from build123d import *

# Parameters (mm, degrees)
SKETCH_1_W      = 450
SKETCH_1_H      = 400
EXTRUDE_1_DEPTH = 50
SKETCH_2_W      = 450
SKETCH_2_H      = 30
EXTRUDE_2_DEPTH = 400
SKETCH_3_W      = 40
SKETCH_3_H      = 40
EXTRUDE_3_DEPTH = 450
SKETCH_4_W      = 40
SKETCH_4_H      = 40
EXTRUDE_4_DEPTH = 450
SKETCH_5_W      = 40
SKETCH_5_H      = 40
EXTRUDE_5_DEPTH = 450
SKETCH_6_W      = 40
SKETCH_6_H      = 40
EXTRUDE_6_DEPTH = 450


with BuildPart() as part:
    # Sketch 1 → Extrude 1 (new body)
    with BuildSketch(Plane.XY):
        Rectangle(SKETCH_1_W, SKETCH_1_H)
    extrude(amount=EXTRUDE_1_DEPTH)

    # Sketch 2 → Extrude 2 (add)
    with BuildSketch(Plane(origin=(0, 0, 0), x_dir=(-1, 0, 0), z_dir=(0, 0, -1))):
        Rectangle(SKETCH_2_W, SKETCH_2_H)
    extrude(amount=EXTRUDE_2_DEPTH)

    # Sketch 4 → Extrude 4 (add)
    with BuildSketch(Plane.XY):
        with Locations((-180, 150)):
            Rectangle(SKETCH_4_W, SKETCH_4_H)
    extrude(amount=EXTRUDE_4_DEPTH)



with BuildPart() as body_2:
    # Sketch 3 → Extrude 3 (new body)
    with BuildSketch(Plane.XZ.offset(15)):
        with Locations((180, 150)):
            Rectangle(SKETCH_3_W, SKETCH_3_H)
    extrude(amount=EXTRUDE_3_DEPTH)


with BuildPart() as part_1:
    add(part.part)

    add(body_2.part)  # Extrude 5 merges body 2
    # Sketch 5 → Extrude 5 (add)
    with BuildSketch(Plane.XY):
        with Locations((180, -150)):
            Rectangle(SKETCH_5_W, SKETCH_5_H)
    extrude(amount=EXTRUDE_5_DEPTH)

    # Sketch 6 → Extrude 6 (add)
    with BuildSketch(Plane.XY):
        with Locations((-180, -150)):
            Rectangle(SKETCH_6_W, SKETCH_6_H)
    extrude(amount=EXTRUDE_6_DEPTH)


solid = part_1.part
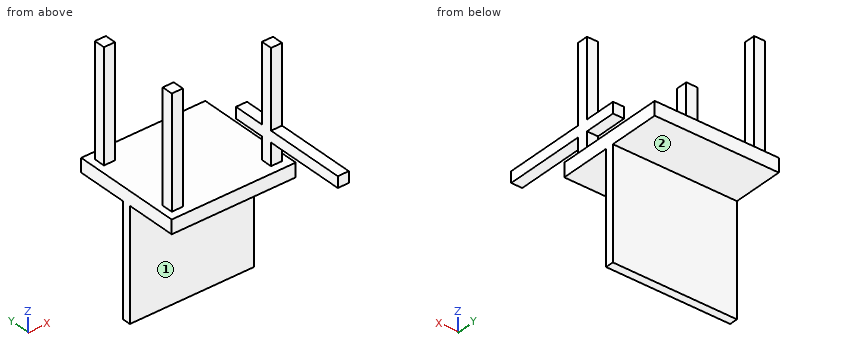
Can you work these out from the model? Positions are in its coordinate system, mm. Face numbers are marked on the shaded views. A direction names the side the tool comes from. Coordinates: 2 decimals unless noted, no trailing zeros. Order: outer loops, then holes, each group sorted by start corner. A loop starts at its lowest first (then second) coordinate and runs counter-clockwise, first axis right, second up. Notation, with made-up numbers: M -22.5,82 L 22.5,82 A15 cw 22.5,89 Z; hole C -35.75,89 d6. An arc over 180 degrees is marked long. Write item = value, one per line.
(1) Suppose I cut it at B-B on z = 252. Please give me the cut outline in (x, y).
Results are:
outline = M -200,-170 L -160,-170 L -160,-130 L -200,-130 Z; M -200,130 L -160,130 L -160,170 L -200,170 Z; M 160,-170 L 200,-170 L 200,-130 L 160,-130 Z
(2) Suppose I cut it at D-D on y = -147.5. Please give me the cut outline in (x, z), plus the area to 3 significant figures.
Results are:
outline = M -225,0 L 225,0 L 225,50 L 200,50 L 200,450 L 160,450 L 160,50 L -160,50 L -160,450 L -200,450 L -200,50 L -225,50 Z
area = 54,500 mm2
(3) I need wall thicknesses on line 1 along X through (y, z) = (-154, 200.5); line 2 along Z through (x, y) = (-7.5, -143.5); line 3 along Z through (x, y) = (105, 3). Which ranges of each line are inside material? Lowest first, please. Write a range as [from, to].
Results are:
line_1 = [-200, -160], [160, 200]
line_2 = [0, 50]
line_3 = [-400, 50]
(4) For pin 1 Ø12 at (x, z) = (176, 304) entering from -Y; pin 2 Ø1 at (x, z) = (-114.5, -145.5) entering from -Y; pin 3 Ø20 at (x, z) = (-184.5, 294.5) entering from +Y, each with a flat end and sliding along its axis, tell me the tip position at first contact or that it passes through.
Results are:
pin_1 = -170
pin_2 = -15
pin_3 = 170
(5) Suppose I cut it at C-C on x = 35. Please give me the cut outline in (y, z), plus the area to 3 significant figures.
Results are:
outline = M -200,0 L -15,0 L -15,-400 L 15,-400 L 15,0 L 200,0 L 200,50 L -200,50 Z
area = 32,000 mm2
(6) Suppose I cut it at A-A on y = -66. Please give me the cut outline in (x, z).
Results are:
outline = M -225,0 L 225,0 L 225,50 L -225,50 Z; M 160,130 L 200,130 L 200,170 L 160,170 Z
(7) For the marked faces 1 and 2, which set-ups out of +Z, -Z, +X, -X, +Y, -Y let a thin tool reach every point of the face, with its end or its side?
Results are:
face_1 = -Z, +X, -X, -Y
face_2 = -Z, +X, -X, +Y
